Geometry check sheet. Reference: the model listing, model coordinates, mm. A direction names the side the tool comes from. Give positions to 0.01 mm unless a question says otherwise; leave off trailing zeros. Order: outer loops, then holes, each group sorted by start corner. A loop starts at its lowest first (then second) coordinate and runs counter-clockwise, first axis right, second up.
Autodesk Inventor part; units mm, degrees
ref_plane "YZ Plane" through (0, 0, 0) normal (1, 0, 0) x (0, 1, 0)
ref_plane "XZ Plane" through (0, 0, 0) normal (0, 1, 0) x (-1, 0, 0)
ref_plane "XY Plane" through (0, 0, 0) normal (0, 0, 1) x (1, 0, 0)
ref_plane "Work Plane1" through (0, 0, 0) normal (0, 0, 1) x (1, 0, 0)
sketch "Sketch1" plane through (0, 0, 0) normal (0, 0, 1) x (1, 0, 0)
  line L0 (-849.45, 463.2386) -> (11.35, 463.2386)
  line L1 (11.35, 463.2386) -> (11.35, 863.2386)
  line L2 (11.35, 863.2386) -> (-849.45, 863.2386)
  line L3 (-849.45, 863.2386) -> (-849.45, 463.2386)
  line L4 (-844.45, 1225.4) -> (-844.45, -25.4)
  line L5 (6.35, -25.4) -> (6.35, 1225.4)
  point P0 (0, 0)
  point P1 (6.35, 463.2386)
  point P2 (6.35, 863.2386)
  point P3 (-844.45, 863.2386)
  point P4 (-844.45, 463.2386)
  dimension "d1" = 400
  dimension "d2" = 5
  dimension "d3" = 5
extrude "Plate1" add sketch "Sketch1" along normal blind 0.5 contours L4 L2 L5 L0
sketch "Sketch2" plane through (5.85, 863.2386, 0.5) normal (1, 0, 0) x (0, 1, 0)
  line L0 (-400, 0) -> (0, 0)
  line L1 (0, 0) -> (0, 25)
  line L2 (0, 25) -> (-400, 25)
  line L3 (-400, 25) -> (-400, 0)
edge flange "Flange1" height 25 angle 90 thickness 0.5 bend radius 0.5 thickness toward (1, 0, 0) relief tear relief width 0.5 relief depth 0.25 corner gap 0.5 corner form 0 edges at (6.35, 663.2386, 0.5) (-844.45, 663.2386, 0.5) wall of the first edge with corners at (5.85, 463.2386, 0.5) (5.85, 863.2386, 0.5) (5.85, 863.2386, -24.5) (5.85, 463.2386, -24.5)
bend "Bend1"
corner "Corner1"
move faces "Move1" translate (0, 320.75, 0) faces at (-560.5167, 463.2386, 0.3333) (-277.5833, 863.2386, 0.3333)
equation "\"d4\" = Thickness"
equation "\"d5\" = BendReliefWidth"
equation "\"d6\" = BendReliefDepth"
equation "\"d7\" = MinimumRemnant"
equation "\"d8\" = TransitionRadius"
equation "\"d11\" = BendRadius"
equation "\"d12\" = CornerReliefSize"
equation "\"d13\" = GapSize"
equation "\"d14\" = JacobiRadiusSize"
equation "\"BendRadius\" = Thickness"
equation "\"BendReliefWidth\" = Thickness"
equation "\"BendReliefDepth\" = 0.5 * Thickness"
equation "\"CornerReliefSize\" = 4 * Thickness"
equation "\"MinimumRemnant\" = 2 * Thickness"
equation "\"TransitionRadius\" = BendRadius"
equation "\"JacobiRadiusSize\" = BendRadius"
equation "\"GapSize\" = Thickness"
properties part number "ENGINE_BASE" material "Stainless Steel, Austenitic"
Item 1: Set-up check for faces 1 (the flat face through (-844.45, 987, -13)), 2 (the flat face through (-843.95, 987, -12)): record each of +Z, -Z, +X, -X, +Y, -Y from which the full face is reachable in a straight line by a thin tool's end or side.
Reported:
face 1: +Z, -Z, -X, +Y, -Y
face 2: -Z, +Y, -Y
Item 2: Gauge pin test, flat end, axial feed: pin 1 (4 mm diameter, centred on x = -196, y = 855.5, fed in from -Z). Record the tip position at first contact, or that the pin passes through.
Reported:
pin 1: stops at z = 0
Item 3: Scan lines: L1, parallel to X at y = 992, z = -9; L2, parallel to Z at x = -798, y = 1061. Record each from-to range of solid material in increasing order.
Reported:
L1: x = -844.45 to -843.95, 5.85 to 6.35
L2: z = 0 to 0.5
Item 4: Sectioned sample at A-A (z = -9). Enter the section's corners in (x, y).
Reported:
outline: (-844.45, 783.99) - (-843.95, 783.99) - (-843.95, 1183.99) - (-844.45, 1183.99) - close; (5.85, 783.99) - (6.35, 783.99) - (6.35, 1183.99) - (5.85, 1183.99) - close
Item 5: Sectioned sample at B-B (y = 1106). Enter the section's corners in (x, z).
Reported:
outline: (-844.45, -24.5) - (-843.95, -24.5) - (-843.95, -0.5) arc R0.5 cw to (-843.45, 0) - (5.35, 0) arc R0.5 cw to (5.85, -0.5) - (5.85, -24.5) - (6.35, -24.5) - (6.35, -0.5) arc R1 ccw to (5.35, 0.5) - (-843.45, 0.5) arc R1 ccw to (-844.45, -0.5) - close
Item 6: Draft check along X on faces 3 (the flat face through (5.85, 981, -12)), 4 (the flat face through (-425, 987, 0.5)), 5 (the flat face through (-425, 987, 0)), 6 (the flat face through (6.35, 981, -13)). Enter one of: released by +X, released by -X, zero draft, split by the parting line, or undercut.
Reported:
face 3: undercut
face 4: zero draft
face 5: undercut
face 6: released by +X
Item 7: Sectioned sample at C-C (x = -403.5). Enter the section's corners in (y, z).
Reported:
outline: (783.99, 0) - (1183.99, 0) - (1183.99, 0.5) - (783.99, 0.5) - close
